Geometry: final body of the model. Coordinates: model frame, mm. Face numbers are marked on the shaded views. A direction names the side the tool comes from. Coordinates: 2 decimals unless noted, no trailing zeros. Order: outer loops, then holes, each group sorted by start corner. A loop starts at its lowest first (then second) coordinate and runs counter-clockwise, first axis right, second up. Notation, with made-up numbers: (69, 70) -> (99, 70) arc R31 ccw to (99, 96) -> close; hole circle Ø7 at (69, 87). An arc over 180 degrees is marked (long way). Answer in a Markdown table with one row per item. Add a question column.
1) Set-up query: the marked faces 5 and 6. Return all of +Z, -Z, +X, -X, +Y, -Y with unobstructed straight access to the full face (end or side cutting, diameter ignored); none if empty.
2) Section query A-A on y = -53.5. Return the cut outline in (x, z).
3) Ray query, line 1 (X direction, y = -56.75, z = -1.5); line 2 (Z direction, x = 0, y = -53.5); line 3 (X direction, y = -55, z = 1.25). Return the intervals inside material, ascending. Write a range as from..to.
4) Section query C-C on z = 1.25. Count the separate pieces of the cut face and the enclosed holes in it, then the cut area to 3 significant figures.
5) Pull-direction query (Z, two-part tool) for the marked faces 1, 2, 3 and 4; classes: +Z half, -Z half, draft (parallel to the pull), parting line (faces both ways), or undercut.
6) Section query B-B on x = 9.15. Return the cut outline in (y, z), then the cut area to 3 significant figures.
7) Section query D-D on x = 13. Return the cut outline in (y, z).
```python
from build123d import *

# Parameters (mm, degrees)
SKETCH005_R     = 1.65
PAD003_DEPTH    = 12
SKETCH006_R     = 2.15
POCKET004_DEPTH = 20
CHAMFER002_SIZE = 0.3
FILLET002_R     = 1.5
SKETCH007_R     = 1.6
POCKET005_DEPTH = 0.4
CHAMFER003_SIZE = 0.3


with BuildPart() as part:
    # Sketch005 → Pad003 (new body)
    with BuildSketch(Plane.XZ):
        with BuildLine():
            ThreePointArc((0, 4.65), (-4.65, 0), (0, -4.65))
            Line((18.300003, -4.65), (0, -4.65))
            ThreePointArc((18.300003, -4.65), (22.95, 2e-06), (18.3, 4.65))
            Line((0, 4.65), (18.3, 4.65))
        make_face()
        Circle(SKETCH005_R, mode=Mode.SUBTRACT)
        with Locations((18.3, 0)):
            Circle(SKETCH005_R, mode=Mode.SUBTRACT)
    extrude(amount=PAD003_DEPTH)

    # Sketch006 (on Face2 of Pad003) → Pocket004 (cut)
    with BuildSketch(Plane(origin=(0, 0, 4.65), x_dir=(-1, 0, 0), z_dir=(0, 0, 1))):
        with Locations((-9.15, 6)):
            Circle(SKETCH006_R)
    extrude(amount=-POCKET004_DEPTH, mode=Mode.SUBTRACT)

    # Chamfer002
    chamfer002_edges = [part.edges().sort_by_distance(p)[0] for p in [
        (-1.65, -12, 0),
        (11.3, -6, 4.65),
        (16.65, -12, 0),
        (16.65, 0, 0),
        (-1.65, 0, 0),
    ]]
    chamfer(chamfer002_edges, length=CHAMFER002_SIZE)

    # Fillet002
    fillet002_edges = [part.edges().sort_by_distance(p)[0] for p in [
        (-4.65, 0, 0),
        (-4.65, -12, 0),
    ]]
    fillet(fillet002_edges, radius=FILLET002_R)

    # Sketch007 (on Face13 of Fillet002) → Pocket005 (cut)
    with BuildSketch(Plane.XZ.offset(12)):
        with Locations((9.15, 0)):
            Circle(SKETCH007_R)
    extrude(amount=-POCKET005_DEPTH, mode=Mode.SUBTRACT)

    # Chamfer003
    chamfer003_edges = [part.edges().sort_by_distance(p)[0] for p in [
        (7.55, -12, 0),
    ]]
    chamfer(chamfer003_edges, length=CHAMFER003_SIZE)


with BuildPart() as part_1:
    # Body002 placement: moved
    add(part.part.moved(Location((0, -47.5, 0))))


solid = part_1.part
```
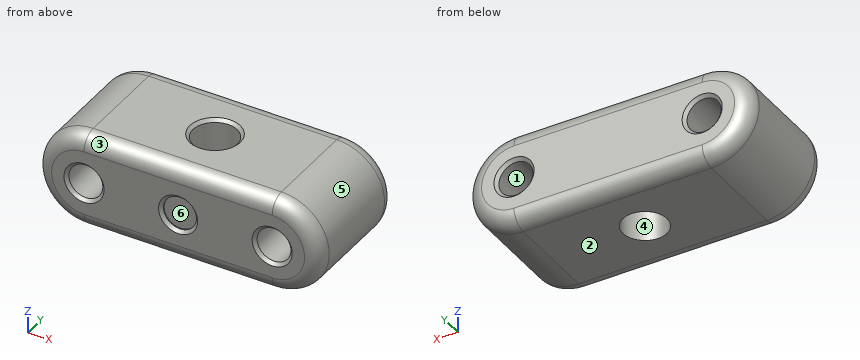
Result:
| question | item | result |
|---|---|---|
| 1 | face 5 | +X, +Y, -Y |
| 1 | face 6 | -Y |
| 2 | outline | (0, -4.65) -> (7, -4.65) -> (7, 4.35) -> (6.7, 4.65) -> (0, 4.65) arc R4.65 ccw to start; (11.3, -4.65) -> (18.3, -4.65) arc R4.65 ccw to (18.3, 4.65) -> (11.6, 4.65) -> (11.3, 4.35) -> close; hole circle Ø3.3 at (0, 0); hole circle Ø3.3 at (18.3, 0) |
| 3 | line 1 | -4.4..-0.69, 0.69..17.61, 18.99..22.7 |
| 3 | line 2 | -4.65..-1.65, 1.65..4.65 |
| 3 | line 3 | -4.48..-1.08, 1.08..7.61, 10.69..17.22, 19.38..22.78 |
| 4 | separate pieces | 3 |
| 4 | enclosed holes | 1 |
| 4 | area | 257 mm2 |
| 5 | face 1 | undercut |
| 5 | face 2 | -Z half |
| 5 | face 3 | +Z half |
| 5 | face 4 | draft |
| 6 | outline | (-59.5, -3.15) arc R1.5 ccw to (-58, -4.65) -> (-55.65, -4.65) -> (-55.65, 4.35) -> (-55.95, 4.65) -> (-58, 4.65) arc R1.5 ccw to (-59.5, 3.15) -> (-59.5, 1.9) -> (-59.2, 1.6) -> (-59.1, 1.6) -> (-59.1, -1.6) -> (-59.2, -1.6) -> (-59.5, -1.9) -> close; (-51.35, -4.65) -> (-49, -4.65) arc R1.5 ccw to (-47.5, -3.15) -> (-47.5, 3.15) arc R1.5 ccw to (-49, 4.65) -> (-51.05, 4.65) -> (-51.35, 4.35) -> close |
| 6 | area | 68.2 mm2 |
| 7 | outline | (-59.5, -3.15) arc R1.5 ccw to (-58, -4.65) -> (-49, -4.65) arc R1.5 ccw to (-47.5, -3.15) -> (-47.5, 3.15) arc R1.5 ccw to (-49, 4.65) -> (-58, 4.65) arc R1.5 ccw to (-59.5, 3.15) -> close |
